Verification items for the finished model (mm, model axes). Round coordinates to 2 decimals unless told otherwise and drop trailing zeros. Write each loop counter-clockwise with the first axis right and the second up, starting at its lowest first coordinate (ties: lowest second). Pieces come first, ordered by that corner, then holes. Notation, with made-up numbers: M -13,27.5 L 26,27.5 A23 ccw 26,46.5 Z; hole C -27,-35 d7. An arc over 180 degrees is marked long. One line per question, with ' | ' between items.
from build123d import *

# Parameters (mm, degrees)
PAD_DEPTH     = 2.5
SKETCH001_R   = 3.5
SKETCH001_R_2 = 2.8
POCKET_DEPTH  = 2.501


with BuildPart() as part:
    # Sketch → Pad (new body)
    with BuildSketch(Plane.XY):
        with BuildLine():
            Line((-9, 30), (9, 30))
            ThreePointArc((12, 27), (11.12132, 29.12132), (9, 30))
            Line((12, 27), (12, -27))
            ThreePointArc((9, -30), (11.12132, -29.12132), (12, -27))
            Line((9, -30), (-9, -30))
            ThreePointArc((-12, -27), (-11.12132, -29.12132), (-9, -30))
            Line((-12, -27), (-12, 27))
            ThreePointArc((-9, 30), (-11.12132, 29.12132), (-12, 27))
        make_face()
    extrude(amount=PAD_DEPTH)

    # Sketch001 (on Face10 of Pad) → Pocket (cut, through all)
    with BuildSketch(Plane.XY.offset(2.5)):
        with Locations((0, 23)):
            Circle(SKETCH001_R)
        with Locations((0, 13)):
            Circle(SKETCH001_R)
        with Locations((0, -13)):
            Circle(SKETCH001_R)
        with Locations((0, -23)):
            Circle(SKETCH001_R)
        with Locations((0, -3)):
            Circle(SKETCH001_R)
        with Locations((-7, 18)):
            Circle(SKETCH001_R_2)
        with Locations((7, 18)):
            Circle(SKETCH001_R_2)
        with Locations((-7, -8)):
            Circle(SKETCH001_R_2)
        with Locations((7, -8)):
            Circle(SKETCH001_R_2)
        with Locations((-7, -18)):
            Circle(SKETCH001_R_2)
        with Locations((7, -18)):
            Circle(SKETCH001_R_2)
    extrude(amount=-POCKET_DEPTH, mode=Mode.SUBTRACT)


solid = part.part
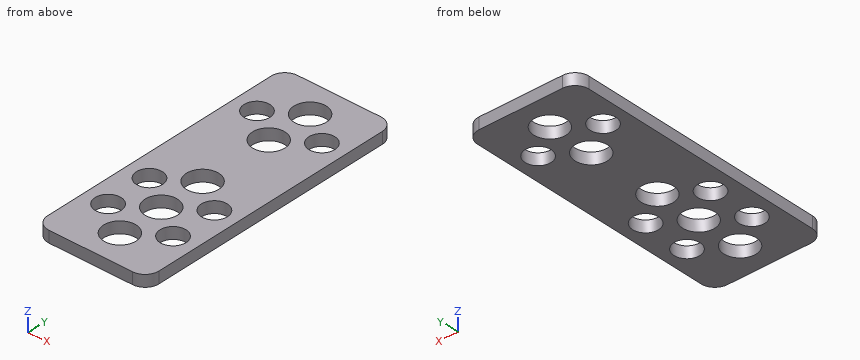
1. Section check A-A, the plane y = -18. Record the cut outline in (x, z).
Results:
outline: M -12,0 L -9.8,0 L -9.8,2.5 L -12,2.5 Z; M -4.2,0 L 4.2,0 L 4.2,2.5 L -4.2,2.5 Z; M 9.8,0 L 12,0 L 12,2.5 L 9.8,2.5 Z
2. Thickness scan on line 1 (Y direction, x = 0, z = 1.75); line 2 (Y direction, x = -7, z = 1.6); line 3 (Y direction, x = -6.25, z = 1.7). Record the ranges inside material, lowest first.
Results:
line 1: y = -30 to -26.5, -19.5 to -16.5, -9.5 to -6.5, 0.5 to 9.5, 16.5 to 19.5, 26.5 to 30 | line 2: y = -30 to -20.8, -15.2 to -10.8, -5.2 to 15.2, 20.8 to 30 | line 3: y = -30 to -20.7, -15.3 to -10.7, -5.3 to 15.3, 20.7 to 30
3. Section check B-B, the plane x = -7. Record the cut outline in (y, z), then the cut area to 3 significant figures.
Results:
outline: M -30,0 L -20.8,0 L -20.8,2.5 L -30,2.5 Z; M -15.2,0 L -10.8,0 L -10.8,2.5 L -15.2,2.5 Z; M -5.2,0 L 15.2,0 L 15.2,2.5 L -5.2,2.5 Z; M 20.8,0 L 30,0 L 30,2.5 L 20.8,2.5 Z | area: 108 mm2
4. Section check C-C, the plane y = 13. Record the cut outline in (x, z), then the cut area to 3 significant figures.
Results:
outline: M -12,0 L -3.5,0 L -3.5,2.5 L -12,2.5 Z; M 3.5,0 L 12,0 L 12,2.5 L 3.5,2.5 Z | area: 42.5 mm2
5. Section check D-D, the plane z = 2. Count the separate pieces of the cut face and the enclosed holes in it, then the cut area to 3 significant figures.
Results:
separate pieces: 1 | enclosed holes: 11 | area: 1,090 mm2
6. Go/stop test with a flat-tipped pin: P1, Ø3.5, axis at x = -7, y = -18, coming from the -Z side. Record where the tip stops, or that it passes through.
Results:
P1: passes through
